Check sheet for the drawn part. Datum: minimum x, y, z corner. Units: mm. A direction names the side the tool comes from. Give positions to 0.01 mm unless a question says otherwise; leave off trailing zeros. Order: outer loops, then holes, each group sorted by start corner. A loop starts at its lowest first (then second) coordinate and runs counter-clockwise, first axis right, second up.
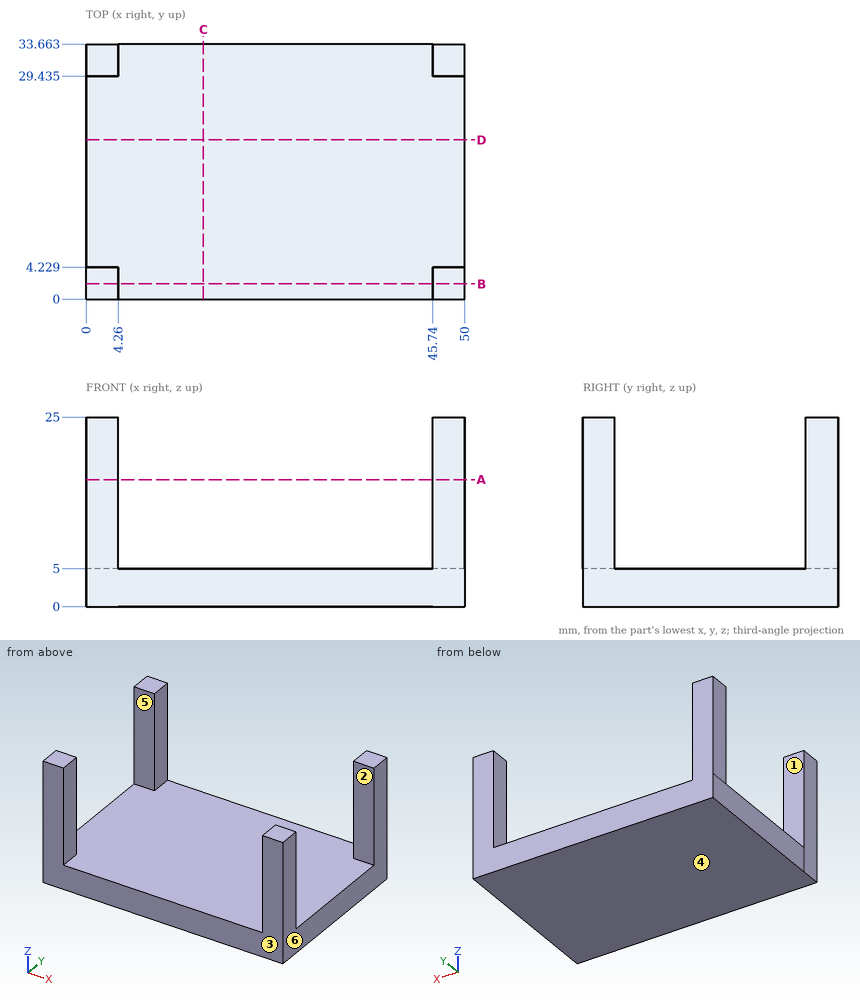
Q1. Sectioned sample at D-D, the plane y = 21. Record the cut outline in (x, z), plus the area to 3 significant figures.
Q2. Draft check along Y on the marked faces 1, 2, 3 and 4. Enter one of: pulls with the +Y half, pulls with the -Y half, needs draft (parallel to the pull), parting line crosses it, or undercut.
Q3. Tool access check on the marked faces 5 and 6. Record the directions out of +Z, -Z, +X, -X, +Y, -Y that give a thin tool (end or side, any length) a straight path to the whole face; none if there is none.
Q4. Go/stop test with a flat-tipped pin: P1, Ø1, axis at x = 39.5, y = 16.5, coming from the +Z side. Record where the tip stops, or that it passes through.
Q5. Material ranges on line 1 (X direction, y = 31, z = 9.25); line 2 (Y direction, x = 4, z = 7.25) (1 decimal); line 3 (Z direction, x = 12, y = 10), recorded low to high.
Q6. Sectioned sample at A-A, the plane z = 16.75. Record the cut outline in (x, y) (1 decimal).
Q7. Sectioned sample at C-C, the plane x = 15.5. Record the cut outline in (y, z), plus the area to 3 significant figures.
Q8. Sectioned sample at B-B, the plane y = 2. Record the cut outline in (x, z).
Filled in:
1. outline: (0, 0) - (50, 0) - (50, 5) - (0, 5) - close
1. area: 250 mm2
2. face 1: undercut
2. face 2: undercut
2. face 3: pulls with the -Y half
2. face 4: needs draft
3. face 5: +Z, +X, -X
3. face 6: +Z, -Z, +X, +Y, -Y
4. P1: stops at z = 5
5. line 1: x = 0 to 4.26, 45.74 to 50
5. line 2: y = 0 to 4.2, 29.4 to 33.7
5. line 3: z = 0 to 5
6. outline: (0, 0) - (4.3, 0) - (4.3, 4.2) - (0, 4.2) - close; (0, 29.4) - (4.3, 29.4) - (4.3, 33.7) - (0, 33.7) - close; (45.7, 0) - (50, 0) - (50, 4.2) - (45.7, 4.2) - close; (45.7, 29.4) - (50, 29.4) - (50, 33.7) - (45.7, 33.7) - close
7. outline: (0, 0) - (33.66, 0) - (33.66, 5) - (0, 5) - close
7. area: 168 mm2
8. outline: (0, 0) - (50, 0) - (50, 25) - (45.74, 25) - (45.74, 5) - (4.26, 5) - (4.26, 25) - (0, 25) - close
